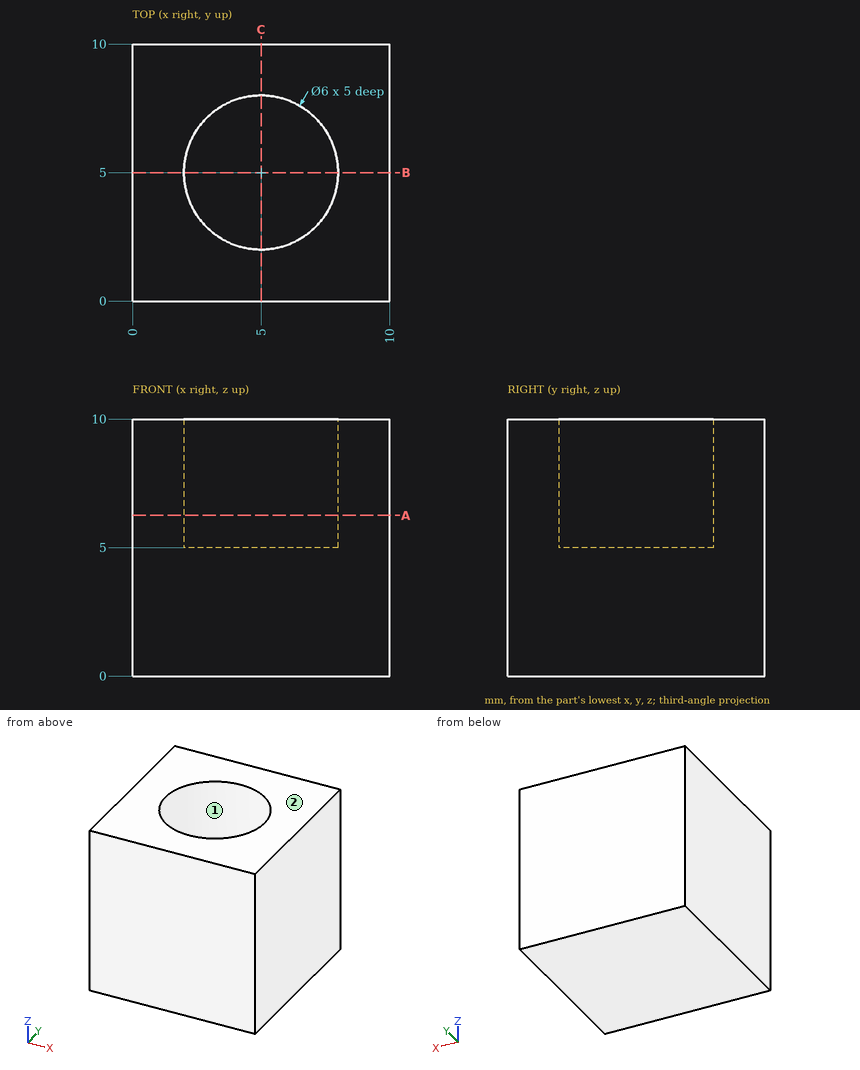
Could you check a few things on this drawing? It's one solid part, dimensions in mm from its lowest x, y, z. A direction names the side the tool comes from. Round coordinates to 2 decimals unless told otherwise and drop trailing zeros. Write each loop counter-clockwise with the first axis right and the second up, starting at its lowest first coordinate (ties: lowest second). Pieces come first, ordered by that corner, then holes. Notation, with made-up numbers: (16.5, 86.5) -> (44.5, 86.5) arc R19 cw to (44.5, 94.5) -> close; hole circle Ø3 at (-18, -28). An arc over 180 degrees is marked (long way). Use one line per item in the form item = value. Start each with the question number.
Q1. If I drill on probe 1 along X at (y, z) = (5, 8.2); probe 2 along X at (y, z) = (3, 8.25), over which ranges is the centre line in solid material (lowest first)? Write a range as [from, to].
Q2. Imagine slicing it at B-B (y = 5). Please give me the cut outline in (x, z).
Q3. I'm going to push a flat-ended pin straight in: P1, Ø1, axis at x = 6, y = 4.5, coming from the +Z side. Where does the tip first touch, or does it pass through?
Q4. Imagine slicing it at A-A (z = 6.25). Please give me the cut outline in (x, y).
Q5. Which directions (+Z, -Z, +X, -X, +Y, -Y) give clear straight access to the entire face, cutting with the end or side of a thin tool? Please do the marked faces 1 and 2.
Worked out:
q1.probe_1 = [0, 2], [8, 10]
q1.probe_2 = [0, 2.76], [7.24, 10]
q2.outline = (0, 0) -> (10, 0) -> (10, 10) -> (8, 10) -> (8, 5) -> (2, 5) -> (2, 10) -> (0, 10) -> close
q3.P1 = 5
q4.outline = (0, 0) -> (10, 0) -> (10, 10) -> (0, 10) -> close; hole circle Ø6 at (5, 5)
q5.face_1 = +Z
q5.face_2 = +Z, +X, -X, +Y, -Y
